Check sheet for the drawn part. Datum: minimum x, y, z corner. Units: mm. A direction names the side the tool comes from. Coordinates: 2 decimals unless noted, no trailing zeros. Order: outer loops, then holes, each group sorted by start corner. A loop starts at its lowest first (then second) coordinate and runs counter-clockwise, first axis right, second up. Notation, with made-up numbers: (32, 79.25) -> (88, 79.25) arc R35 ccw to (88, 115.25) -> close; hole circle Ø11 at (1.25, 71). An arc over 180 degrees is marked (long way). Answer as CSV lines item,"result".
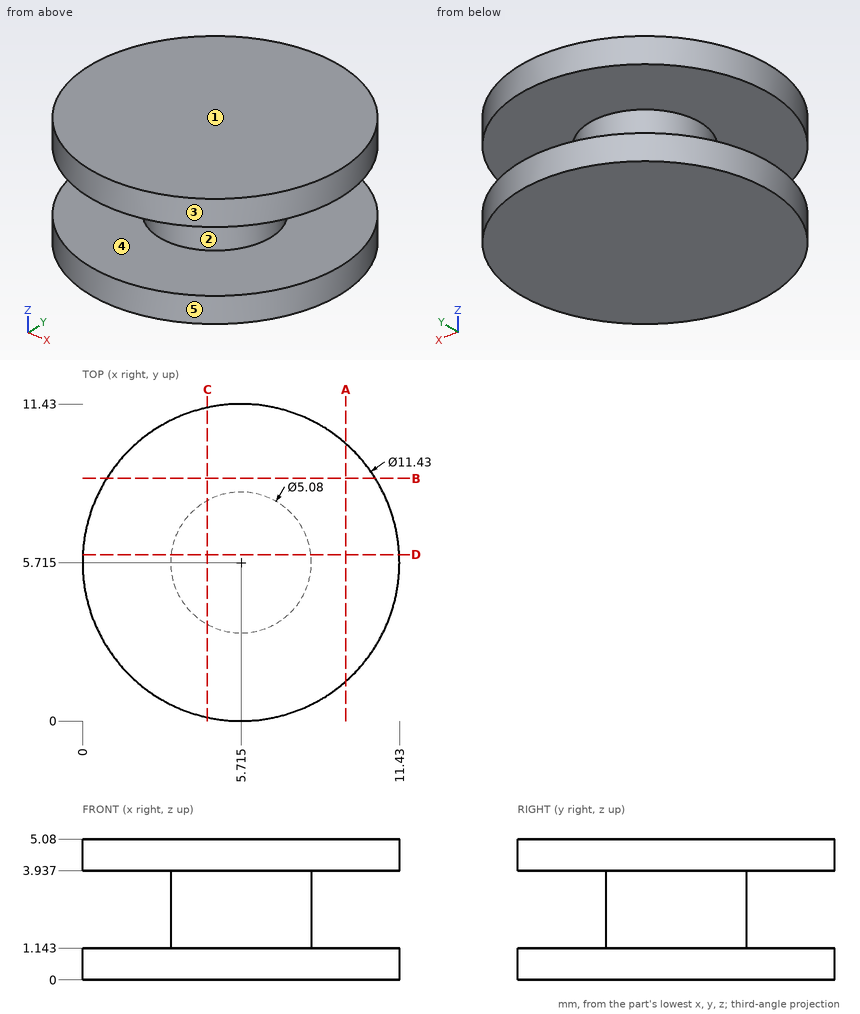
Item 1: Section check C-C, the plane x = 4.5. Record the boundary of the cut face in (y, z), plus the area to 3 significant figures.
Answer list:
outline,"(0.13, 0) -> (11.3, 0) -> (11.3, 1.14) -> (7.95, 1.14) -> (7.95, 3.94) -> (11.3, 3.94) -> (11.3, 5.08) -> (0.13, 5.08) -> (0.13, 3.94) -> (3.48, 3.94) -> (3.48, 1.14) -> (0.13, 1.14) -> close"
area,"38.0 mm2"
Item 2: Section check D-D, the plane y = 6. Record the boundary of the cut face in (x, z).
Answer list:
outline,"(0.01, 0) -> (11.42, 0) -> (11.42, 1.14) -> (8.24, 1.14) -> (8.24, 3.94) -> (11.42, 3.94) -> (11.42, 5.08) -> (0.01, 5.08) -> (0.01, 3.94) -> (3.19, 3.94) -> (3.19, 1.14) -> (0.01, 1.14) -> close"
Item 3: Section check A-A, the plane x = 9.5. Record the boundary of the cut face in (y, z), plus the area to 3 significant figures.
Answer list:
outline,"(1.43, 0) -> (10, 0) -> (10, 1.14) -> (1.43, 1.14) -> close; (1.43, 3.94) -> (10, 3.94) -> (10, 5.08) -> (1.43, 5.08) -> close"
area,"19.6 mm2"
Item 4: Thickness scan on line 1 (Z direction, x = 3.25, y = 4.25); line 2 (Y direction, x = 6.5, z = 0.2); line 3 (X direction, y = 4, z = 2.05). Record the ranges inside material, lowest first.
Answer list:
line 1,"0 to 1.14, 3.94 to 5.08"
line 2,"0.05 to 11.38"
line 3,"3.84 to 7.59"
Item 5: Section check B-B, the plane y = 8.75. Record the boundary of the cut face in (x, z).
Answer list:
outline,"(0.87, 0) -> (10.56, 0) -> (10.56, 1.14) -> (0.87, 1.14) -> close; (0.87, 3.94) -> (10.56, 3.94) -> (10.56, 5.08) -> (0.87, 5.08) -> close"
Item 6: Release check for a two-part mould opening along Z. For the marked faces 1, 2 and 3 record: +Z half, -Z half, draft (parallel to the pull), parting line (faces both ways), or undercut.
Answer list:
face 1,"+Z half"
face 2,"undercut"
face 3,"draft"
Item 7: Depth check by flat-ended pin: pin 1 Ø1.5 at (x, z) = (1, 4.5) entering from +Y; pin 2 Ø1 at (y, z) = (3, 4.5) entering from -X. Enter the tip coordinate at first touch or a pass-through.
Answer list:
pin 1,"y = 9.83"
pin 2,"x = 0.45"
Item 8: Tool access check on the marked faces 4 and 5. Record the directions out of +Z, -Z, +X, -X, +Y, -Y that give a thin tool (end or side, any length) a straight path to the whole face; none if there is none.
Answer list:
face 4,"none"
face 5,"+Z, -Z"
